```python
from build123d import *

# Parameters (mm, degrees)
BOSS_EXTRUDE1_DEPTH = 15.875
SKETCH3_R           = 6.5
CUT_EXTRUDE1_DEPTH  = 51.8000001


with BuildPart() as part:
    # Sketch2 → Boss-Extrude1 (new body, symmetric)
    with BuildSketch(Plane(origin=(0, 0, 0), x_dir=(0, 0, -1), z_dir=(1, 0, 0))):
        with BuildLine():
            Line((-38.1, -5.601130621), (-38.1, 45.198869379))
            Line((-38.1, 45.198869379), (38.1, 45.198869379))
            Line((38.1, 45.198869379), (38.1, 3.798196304))
            add(Edge.make_bspline(
                [(-38.1, -5.601130621), (-0.21894309, 0.874475249), (38.1, 3.798196304)],
                knots=[0, 0, 0, 1, 1, 1], degree=2))
        make_face()
    extrude(amount=BOSS_EXTRUDE1_DEPTH, both=True)

    # Sketch3 → Cut-Extrude1 (cut, through all)
    with BuildSketch(Plane(origin=(0, 45.198869379, 0), x_dir=(1, 0, 0), z_dir=(0, 1, 0))):
        with BuildLine():
            Line((0, -38.1), (15.875, -38.1))
            Line((15.875, -38.1), (15.875, -2.65e-07))
            ThreePointArc((15.875, -2.65e-07), (12.001057449, -20.2782212), (0.924852299, -37.700372463))
            ThreePointArc((0.924852299, -37.700372463), (0.503749428, -37.995820104), (0, -38.1))
        make_face()
        with BuildLine():
            ThreePointArc((0.924852299, 37.700372463), (12.001057547, 20.278220954), (15.875, -2.65e-07))
            Line((15.875, -2.65e-07), (15.875, 38.1))
            Line((15.875, 38.1), (0, 38.1))
            ThreePointArc((0, 38.1), (0.503749428, 37.995820104), (0.924852299, 37.700372463))
        make_face()
        with BuildLine():
            Line((-15.875, -38.1), (0, -38.1))
            ThreePointArc((0, -38.1), (-0.503749428, -37.995820104), (-0.924852299, -37.700372463))
            ThreePointArc((-0.924852299, -37.700372463), (-12.001057487, -20.278221106), (-15.875, -6.3e-08))
            Line((-15.875, -6.3e-08), (-15.875, -38.1))
        make_face()
        with BuildLine():
            ThreePointArc((-0.924852299, 37.700372463), (-0.503749428, 37.995820104), (0, 38.1))
            Line((0, 38.1), (-15.875, 38.1))
            Line((-15.875, 38.1), (-15.875, -6.3e-08))
            ThreePointArc((-15.875, -6.3e-08), (-12.00105751, 20.278221048), (-0.924852299, 37.700372463))
        make_face()
        Circle(SKETCH3_R)
    extrude(amount=-CUT_EXTRUDE1_DEPTH, mode=Mode.SUBTRACT)


solid = part.part
```
Verification items for the finished model (mm, model axes). Coordinates: 2 decimals unless noted, no trailing zeros. Write each loop counter-clockwise with the first axis right and the second up, starting at its lowest first coordinate (ties: lowest second). Pieces come first, ordered by that corner, then holes. Notation, with made-up numbers: (11, 28) - (44, 28) arc R29 cw to (44, 65) - close; hole circle Ø7 at (4.25, 81). An arc over 180 degrees is marked (long way). Write item = value, one per line.
Q1. Mould release check, pull along X, two halves, no side actions. Record for faces 1 (the face through (-5.158, 22.508, 3.955)), 2 (the face through (7, 45.199, 1)): released by +X, released by -X, zero draft, split by the parting line, or undercut.
Answer:
face_1 = undercut
face_2 = zero draft
Q2. Cross-section at A-A (y = 36.5). Enter the section's corners in (x, z) (3 decimals).
Answer:
outline = (-0.925, -37.7) arc R1.27 ccw to (0.925, -37.7) arc R55.01 ccw to (0.925, 37.7) arc R1.27 ccw to (-0.925, 37.7) arc R55.01 ccw to start; hole circle Ø13 at (0, 0)
Q3. Go/stop test with flat-tipped pins: pin 1 Ø6 at (x, z) = (12, 2.5) entering from -Y; pin 2 Ø12 at (y, z) = (26.5, 10.5) entering from +X; pin 3 Ø2 at (x, y) = (6, 31) entering from +Z; pin 4 Ø11.5 at (x, z) = (0, 0) entering from -Y. Record where each tip stops, or that it passes through.
Answer:
pin_1 = -0.7
pin_2 = 15.69
pin_3 = 32.84
pin_4 = through
Q4. Material ranges on L1, parallel to Z at x = 0, y = 25; L2, parallel to Z at x = -0.5, y = 8.5; L3, parallel to X at y = 30.5, z = -1.5, recorded low to high. Write a range as from..to.
Answer:
L1 = -38.1..-6.5, 6.5..38.1
L2 = -38..-6.48, 6.48..38
L3 = -15.85..-6.32, 6.32..15.85
